Geometry check sheet. Reference: the model listing, model coordinates, mm. A direction names the side the tool comes from. Coordinates: 2 decimals unless noted, no trailing zeros. Loops run counter-clockwise (first coordinate to the right, second up) from the corner with the lowest first, then second, coordinate; pieces in that order, holes last. Notation, with made-up numbers: (1.25, 23) - (5.25, 23) arc R24 ccw to (5.25, 34) - close; hole circle Ø2 at (64.5, -15). An arc over 180 degrees is marked (long way). Write item = value, one per line. Start each with the question number.
from build123d import *

# Parameters (mm, degrees)
BOSS_EXTRUDE1_DEPTH = 20
CUT_EXTRUDE1_DEPTH  = 17
SKETCH4_W           = 71.5
SKETCH4_H           = 26.25
CUT_EXTRUDE2_DEPTH  = 93.330926563


with BuildPart() as part:
    # Sketch1 → Boss-Extrude1 (new body)
    with BuildSketch(Plane(origin=(0, 0, 0), x_dir=(1, 0, 0), z_dir=(0, 1, 0))):
        with BuildLine():
            Line((-40, -75), (40, -75))
            ThreePointArc((40, -75), (47.071067812, -72.071067812), (50, -65))
            Line((50, -65), (50, 65))
            ThreePointArc((50, 65), (47.071067812, 72.071067812), (40, 75))
            Line((40, 75), (-40, 75))
            ThreePointArc((-40, 75), (-47.071067812, 72.071067812), (-50, 65))
            Line((-50, 65), (-50, -65))
            ThreePointArc((-50, -65), (-47.071067812, -72.071067812), (-40, -75))
        make_face()
    extrude(amount=BOSS_EXTRUDE1_DEPTH)

    # Sketch3 → Cut-Extrude1 (cut)
    with BuildSketch(Plane(origin=(0, 20, 0), x_dir=(1, 0, 0), z_dir=(0, 1, 0))):
        with BuildLine():
            Line((40, 70), (-40, 70))
            ThreePointArc((-40, 70), (-43.535533906, 68.535533906), (-45, 65))
            Line((-45, 65), (-45, -65))
            ThreePointArc((-45, -65), (-43.535533906, -68.535533906), (-40, -70))
            Line((-40, -70), (40, -70))
            ThreePointArc((40, -70), (43.535533906, -68.535533906), (45, -65))
            Line((45, -65), (45, 65))
            ThreePointArc((45, 65), (43.535533906, 68.535533906), (40, 70))
        make_face()
    extrude(amount=-CUT_EXTRUDE1_DEPTH, mode=Mode.SUBTRACT)

    # Sketch4 → Cut-Extrude2 (cut, through all)
    with BuildSketch(Plane.XZ):
        with BuildLine():
            Line((-27.5, -61), (27.5, -61))
            ThreePointArc((27.5, -61), (29.621320344, -60.121320344), (30.5, -58))
            Line((30.5, -58), (30.5, 16))
            ThreePointArc((30.5, 16), (29.621320344, 18.121320344), (27.5, 19))
            Line((27.5, 19), (-27.5, 19))
            ThreePointArc((-27.5, 19), (-29.621320344, 18.121320344), (-30.5, 16))
            Line((-30.5, 16), (-30.5, -58))
            ThreePointArc((-30.5, -58), (-29.621320344, -60.121320344), (-27.5, -61))
        make_face()
        with Locations((0, 50.125)):
            Rectangle(SKETCH4_W, SKETCH4_H)
    extrude(amount=-CUT_EXTRUDE2_DEPTH, mode=Mode.SUBTRACT)


solid = part.part
(1) Sectioned sample at B-B on x = -13.5. Enter the section's corners in (y, z).
(2) Tool access check on faces 4 (the face through (-48, 20, 0)), 5 (the face through (-29.64, 1.48, -60.1)), 6 (the face through (1, 12, -70)). Record the directions out of +Z, -Z, +X, -X, +Y, -Y that give a thin tool (end or side, any length) a straight path to the whole face; none if there is none.
(3) Draft check along Z on faces 1 (the face through (-1, 12, 70)), 2 (the face through (46.99, 9.86, 72.15)), 3 (the face through (47.15, 9.86, -71.99)). Enter one of: pulls with the +Z half, pulls with the -Z half, needs draft (parallel to the pull), parting line crosses it, or undercut.
(4) Depth check by flat-ended pin: pin 1 (12 mm diameter, centred on x = 4, z = -56.5, fed in from +Y). Enter the tip coordinate at first touch or a pass-through.
(5) Sectioned sample at D-D on z = 51. Enter the section's corners in (x, y), plus the area to 4 significant figures.
(6) Sectioned sample at A-A on z = -21. Enter the section's corners in (x, y).
(7) Scan lines: line 1 (Z direction, x = -18, y = 1); line 2 (Z direction, x = 0.5, y = 10); line 3 (X direction, y = 10.25, z = -27.5). Record each from-to range of solid material in increasing order.
(8) Sectioned sample at C-C on y = 4.5. Enter the section's corners in (x, z), plus the area to 3 significant figures.
Working result:
q1.outline = (0, -75) - (20, -75) - (20, -70) - (3, -70) - (3, -61) - (0, -61) - close; (0, 19) - (3, 19) - (3, 37) - (0, 37) - close; (0, 63.25) - (3, 63.25) - (3, 70) - (20, 70) - (20, 75) - (0, 75) - close
q2.face_4 = +Z, -Z, +X, -X, +Y
q2.face_5 = +Y, -Y
q2.face_6 = +Y
q3.face_1 = undercut
q3.face_2 = pulls with the +Z half
q3.face_3 = pulls with the -Z half
q4.pin_1 = 3
q5.outline = (-50, 0) - (-35.75, 0) - (-35.75, 3) - (-45, 3) - (-45, 20) - (-50, 20) - close; (35.75, 0) - (50, 0) - (50, 20) - (45, 20) - (45, 3) - (35.75, 3) - close
q5.area = 255.5 mm2
q6.outline = (-50, 0) - (-30.5, 0) - (-30.5, 3) - (-45, 3) - (-45, 20) - (-50, 20) - close; (30.5, 0) - (50, 0) - (50, 20) - (45, 20) - (45, 3) - (30.5, 3) - close
q7.line_1 = -75 to -61, 19 to 37, 63.25 to 75
q7.line_2 = -75 to -70, 70 to 75
q7.line_3 = -50 to -45, 45 to 50
q8.outline = (-50, -65) arc R10 ccw to (-40, -75) - (40, -75) arc R10 ccw to (50, -65) - (50, 65) arc R10 ccw to (40, 75) - (-40, 75) arc R10 ccw to (-50, 65) - close; hole (-45, -65) arc R5 ccw to (-40, -70) - (40, -70) arc R5 ccw to (45, -65) - (45, 65) arc R5 ccw to (40, 70) - (-40, 70) arc R5 ccw to (-45, 65) - close
q8.area = 2,340 mm2
